Geometry: final body of the model. Coordinates: model frame, mm. A direction names the side the tool comes from. Give positions to 0.01 mm unless a question says otherwise; leave off trailing zeros. Write each loop counter-clockwise with the first axis right and the second up, starting at its lowest first coordinate (ties: lowest second). Pieces come first, ordered by that corner, then holes.
Q1. Pin query (flat end, axial travel): pin 1 Ø3 at (x, z) = (-29, 1) entering from +Y; pin 2 Ø5 at (x, z) = (-14.5, 4.5) entering from +Y; pin 3 Ø8.5 at (x, y) = (-23.5, 27.5) entering from -Z; pin 4 Ø5 at (y, z) = (18, -0.5) entering from -X. Return the tip coordinate at first contact, or that it passes through.
Q2. Section D-D (z = 5). Return the cut outline in (x, y).
Q3. Mould query, pull axis X, two halves, no side actions, for faces 1 (the flat face through (-0.14, 3.78, 0.09)), 2 (the flat face through (-14.903, 24.456, -1.199)), 3 (the flat face through (-25, 4, -6.35)). Classes: +X half, -X half, draft (parallel to the pull), parting line (faces both ways), or undercut.
Q4. Section C-C (z = 2). Return the cut outline in (x, y), plus the area to 3 significant figures.
Q5. Section B-B (z = -5). Return the cut outline in (x, y), plus the area to 3 significant figures.
Q6. Line query: line 1 (Y direction, x = -33.5, z = -2.75); line 2 (Y direction, x = -15, z = -3); line 3 (Y direction, x = -24, z = -0.5). Output: solid intervals per line, ascending.
Q7. Section A-A (z = -2.25). Return the cut outline in (x, y).
Q8. Reachability of faces 4 (the flat face through (-18.66, 5.77, -0.09)), 5 (the flat face through (-5.183, 6.073, -3.131)) from +Z, -Z, +X, -X, +Y, -Y: full face, straight path, thin tool, end or side. Return the list, or none.
from build123d import *

# Parameters (mm, degrees)
F1_DEPTH = 6.35
F2_DEPTH = 6.35
F3_W     = 50.8
F3_H     = 2.54
F4_DEPTH = 7.62
F6_DEPTH = 7.62


with BuildPart() as f1:
    # F0 (on Top) → F1 (new body)
    with BuildSketch(Plane.XY):
        Polygon((-9.9593002213, -19.26124861), (9.9593002213, 27.47085338), (-40.4711874956, 21.3548163761), align=None)
        Polygon((-10.5709039217, -14.2181998383), (-35.7979772966, 19.3629563319), (5.8976937227, 24.4196646526), align=None, mode=Mode.SUBTRACT)
        Polygon((5.8976937227, 24.4196646526), (-35.7979772966, 19.3629563319), (-10.5709039217, -14.2181998383), align=None)
        Polygon((-11.293270497, -8.2618430214), (-30.2784376915, 17.0103657284), (1.1005206928, 20.8158984391), align=None, mode=Mode.SUBTRACT)
        Polygon((1.1005206928, 20.8158984391), (-30.2784376915, 17.0103657284), (-11.293270497, -8.2618430214), align=None)
        Polygon((-11.9048741973, -3.2187942497), (-25.6052274925, 15.0185056841), (-2.9610858058, 17.7647097116), align=None, mode=Mode.SUBTRACT)
    extrude(amount=F1_DEPTH)

    # F0 (on Top) → F2 (join)
    with BuildSketch(Plane.XY):
        Polygon((-9.9593002213, -19.26124861), (9.9593002213, 27.47085338), (-40.4711874956, 21.3548163761), align=None)
        Polygon((-10.5709039217, -14.2181998383), (-35.7979772966, 19.3629563319), (5.8976937227, 24.4196646526), align=None, mode=Mode.SUBTRACT)
        Polygon((1.1005206928, 20.8158984391), (-30.2784376915, 17.0103657284), (-11.293270497, -8.2618430214), align=None)
        Polygon((-11.9048741973, -3.2187942497), (-25.6052274925, 15.0185056841), (-2.9610858058, 17.7647097116), align=None, mode=Mode.SUBTRACT)
    extrude(amount=-F2_DEPTH)

    # F3 (on face) → F4 (join)
    with BuildSketch(Plane(origin=(-3.1389223385, 25.8823457631, 0), x_dir=(-0.9927261362, -0.1203944292, 0), z_dir=(-0.1203944292, 0.9927261362, 0))):
        with Locations((12.2058046598, 5.08)):
            Rectangle(F3_W, F3_H)
    extrude(amount=F4_DEPTH)

    # F5 (on face) → F6 (join)
    with BuildSketch(Plane(origin=(0, 0, 3.81), x_dir=(1, 0, 0), z_dir=(0, 0, -1))):
        Polygon((9.5617578161, -30.7488350816), (-40.8687299009, -24.6327980777), (-41.3885930462, -28.9193895337), (9.0418946707, -35.0354265375), align=None)
    extrude(amount=F6_DEPTH)


solid = f1.part
Computed:
1. pin 1: stops at y = 30.6
1. pin 2: stops at y = 32.48
1. pin 3: stops at z = -6.35
1. pin 4: stops at x = -39.83
2. outline: (-41.39, 28.92) - (-40.47, 21.35) - (-9.96, -19.26) - (9.96, 27.47) - (9.04, 35.04) - close; hole (-25.61, 15.02) - (-11.9, -3.22) - (-2.96, 17.76) - close
3. face 1: +X half
3. face 2: undercut
3. face 3: draft
4. outline: (-41.39, 28.92) - (-40.87, 24.63) - (9.56, 30.75) - (9.04, 35.04) - close; (-40.47, 21.35) - (-9.96, -19.26) - (9.96, 27.47) - close; hole (-25.61, 15.02) - (-11.9, -3.22) - (-2.96, 17.76) - close
4. area: 1,110 mm2
5. outline: (-40.47, 21.35) - (-9.96, -19.26) - (9.96, 27.47) - close; (-30.28, 17.01) - (-11.29, -8.26) - (1.1, 20.82) - close; hole (-35.8, 19.36) - (-10.57, -14.22) - (5.9, 24.42) - close; hole (-25.61, 15.02) - (-11.9, -3.22) - (-2.96, 17.76) - close
5. area: 561 mm2
6. line 1: y = 12.08 to 16.3, 19.64 to 22.2, 25.53 to 29.88
6. line 2: y = -12.55 to -8.32, -3.33 to 0.9, 16.3 to 18.86, 21.89 to 24.44, 27.77 to 32.12
6. line 3: y = -0.57 to 3.66, 8.65 to 12.88, 15.21 to 17.77, 20.79 to 23.35, 26.68 to 31.03
7. outline: (-41.39, 28.92) - (-40.87, 24.63) - (9.56, 30.75) - (9.04, 35.04) - close; (-40.47, 21.35) - (-9.96, -19.26) - (9.96, 27.47) - close; (-30.28, 17.01) - (-11.29, -8.26) - (1.1, 20.82) - close; hole (-35.8, 19.36) - (-10.57, -14.22) - (5.9, 24.42) - close; hole (-25.61, 15.02) - (-11.9, -3.22) - (-2.96, 17.76) - close
8. face 4: +Z, -Z
8. face 5: -Z
